from build123d import *

# Parameters (mm, degrees)
SKETCH7_W           = 27.5
SKETCH7_H           = 27.5
BOSS_EXTRUDE6_DEPTH = 40
SKETCH8_W           = 15.24
SKETCH8_H           = 15.24
CUT_EXTRUDE2_DEPTH  = 12.5
CUT_EXTRUDE3_DEPTH  = 20
SKETCH10_W          = 22.2
SKETCH10_H          = 22.2
SKETCH10_W_2        = 17.7
SKETCH10_H_2        = 17.7
CUT_EXTRUDE4_DEPTH  = 10
CUT_EXTRUDE5_DEPTH  = 12.5


with BuildPart() as part:
    # Sketch7 → Boss-Extrude6 (new body)
    with BuildSketch(Plane(origin=(0, 0, 0), x_dir=(1, 0, 0), z_dir=(0, 1, 0))):
        with Locations((-1.790038454, -39.090727751)):
            Rectangle(SKETCH7_W, SKETCH7_H)
    extrude(amount=BOSS_EXTRUDE6_DEPTH)

    # Sketch8 → Cut-Extrude2 (cut)
    with BuildSketch(Plane(origin=(0, 40, 0), x_dir=(1, 0, 0), z_dir=(0, 1, 0))):
        with Locations((4.339961546, -45.220727751)):
            Rectangle(SKETCH8_W, SKETCH8_H)
    extrude(amount=-CUT_EXTRUDE2_DEPTH, mode=Mode.SUBTRACT)

    # Sketch9 → Cut-Extrude3 (cut)
    with BuildSketch(Plane.XZ):
        Polygon((-10.240038454, 30.640727751), (-10.240038454, 52.840727751), (-15.540038454, 52.840727751), (-15.540038454, 25.340727751), (11.959961546, 25.340727751), (11.959961546, 30.640727751), align=None)
    extrude(amount=-CUT_EXTRUDE3_DEPTH, mode=Mode.SUBTRACT)

    # Sketch10 → Cut-Extrude4 (cut)
    with BuildSketch(Plane.XZ):
        with Locations((0.859961546, 41.740727751)):
            Rectangle(SKETCH10_W, SKETCH10_H)
        with Locations((0.859961546, 41.740727751)):
            Rectangle(SKETCH10_W_2, SKETCH10_H_2, mode=Mode.SUBTRACT)
    extrude(amount=-CUT_EXTRUDE4_DEPTH, mode=Mode.SUBTRACT)

    # Sketch11 → Cut-Extrude5 (cut)
    with BuildSketch(Plane(origin=(0, 40, 0), x_dir=(1, 0, 0), z_dir=(0, 1, 0))):
        Polygon((11.959961546, -34.340727751), (11.959961546, -25.340727751), (-4.564600262, -25.340727751), (-10.557653768, -25.340727751), (-15.540038454, -25.340727751), (-15.540038454, -52.840727751), (-6.540038454, -52.840727751), (-6.540038454, -34.340727751), align=None)
    extrude(amount=-CUT_EXTRUDE5_DEPTH, mode=Mode.SUBTRACT)


solid = part.part
The listing builds one solid part. Answer for the finished solid, in the listing's coordinates (mm). A direction names the side the tool comes from. Round coordinates to 2 decimals unless told otherwise and drop trailing zeros. Write each loop counter-clockwise with the first axis right and the second up, starting at its lowest first coordinate (ties: lowest second). Pieces come first, ordered by that corner, then holes. Notation, with made-up numbers: M 36.25,-8 L 51.25,-8 A13 cw 51.25,-1 Z; hole C 75,33.25 d11. An arc over 180 degrees is marked long. Write each question's results on one line, items separated by ' | '. Start each with the question number.
(1) Each of these flat-tipped pins is pushed along its axis until it touches: P1, Ø5, axis at x = -3.5, y = 6, coming from the +Z side; P2, Ø8, axis at x = -2, y = 15, coming from the -Z side; P3, Ø4, axis at x = 3.5, y = 31.5, coming from the -Z side. Where does it stop, or does it pass through?
(2) For faces 1 (the flat face through (-10.24, 15, 42)), 2 (the flat face through (1, 5, 32.891)), 3 (the flat face through (9.71, 5, 42)), determine the directions among +Z, -Z, +X, -X, +Y, -Y from which every point of the face is accessible in a straight line to the end or side of a thin tool.
(3) The part is cut by section C-C, the plane y = 33.5. Write down the section's boundary in (x, z), and give its area (3 significant figures).
(4) The part is cut by section D-D, the plane x = -8.5. Write down the section's boundary in (y, z), and give its area (3 significant figures).
(5) The part is cut by section B-B, the plane z = 41.5. Write down the section's boundary in (x, y), and give its area (3 significant figures).
(6) The part is cut by section A-A, the plane x = -2.75. Write down the section's boundary in (y, z), and give its area (3 significant figures).
(7) Find the intervals of material crossed by line 1 (Z direction, x = -6.75, y = 3); line 2 (Y direction, x = 8.25, z = 41); line 3 (Z direction, x = 7.5, y = 36), in increasing order.
Worked answers:
1) P1: stops at z = 50.59 | P2: stops at z = 30.64 | P3: stops at z = 34.34
2) face 1: +Z, -Z, -X, -Y | face 2: -Z, +X, -X, -Y | face 3: +Z, -Z, +X, -Y
3) outline: M -6.54,34.34 L 11.96,34.34 L 11.96,37.6 L -3.28,37.6 L -3.28,52.84 L -6.54,52.84 Z | area: 110 mm²
4) outline: M 10,30.64 L 20,30.64 L 20,25.34 L 27.5,25.34 L 27.5,52.84 L 10,52.84 Z | area: 428 mm²
5) outline: M -15.54,20 L -10.24,20 L -10.24,10 L -7.99,10 L -7.99,0 L 9.71,0 L 9.71,10 L 11.96,10 L 11.96,27.5 L -3.28,27.5 L -3.28,40 L -6.54,40 L -6.54,27.5 L -15.54,27.5 Z | area: 646 mm²
6) outline: M 0,32.89 L 10,32.89 L 10,30.64 L 20,30.64 L 20,25.34 L 27.5,25.34 L 27.5,34.34 L 40,34.34 L 40,37.6 L 27.5,37.6 L 27.5,52.84 L 10,52.84 L 10,50.59 L 0,50.59 Z | area: 646 mm²
7) line 1: z = 32.89 to 50.59 | line 2: y = 0 to 27.5 | line 3: z = 34.34 to 37.6
